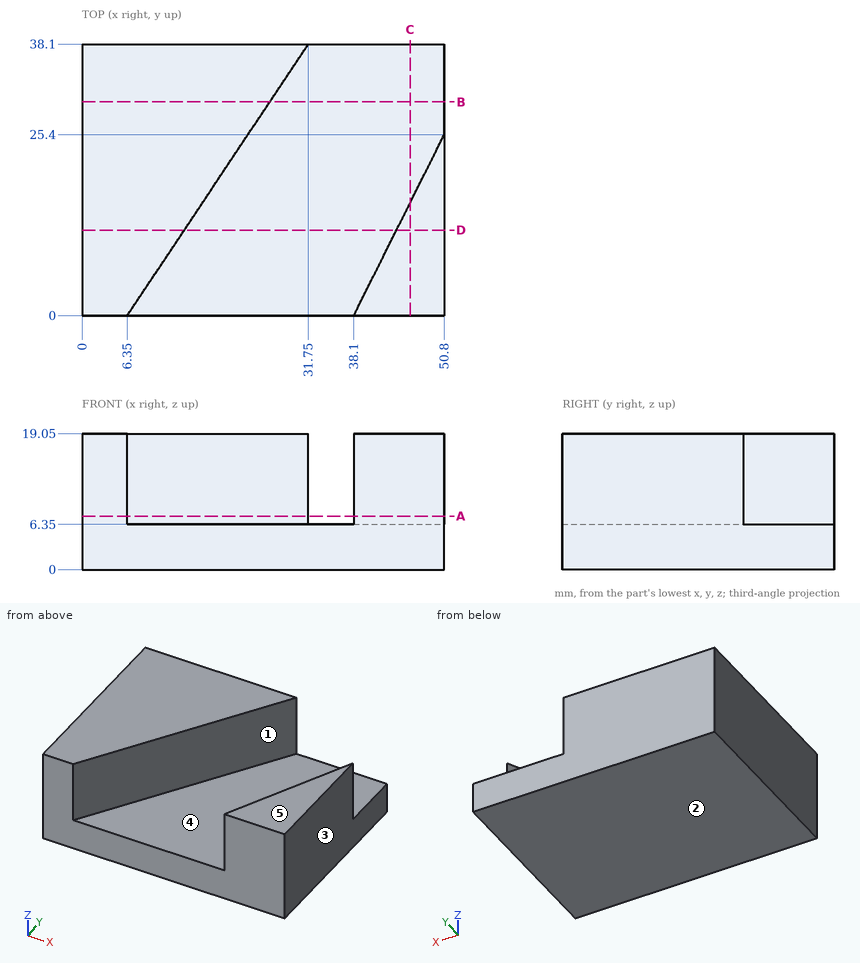
Verification items for this drawing (mm, ordinates from the low corner). A direction names the side the tool comes from. Coordinates: 2 decimals unless noted, no trailing zeros. Order: outer loops, then holes, each group sorted by start corner. A loop starts at its lowest first (then second) coordinate and runs counter-clockwise, first axis right, second up. Notation, with made-up numbers: (-23, 45) - (34, 45) arc R8 ccw to (34, 50) - close; hole circle Ø5 at (17, 70.5). An arc over 180 degrees is marked (long way). Use one line per item in the form item = value.
1. Access from +Z, -Z, +X, -X, +Y, -Y to the whole of each face (thin tool, end or side, straight path). Record for the marked faces 1 and 2.
Here are the results:
face_1 = +Z, -Y
face_2 = -Z, +X, -X, +Y, -Y
2. Gauge pin test, flat ends, axial feed: pin 1 (2 mm diameter, centred on x = 15.5, z = 11, fed in from -Y) (3 decimals); pin 2 (1.5 mm diameter, centred on x = 30.5, z = 9, fed in from -Y). Record the tip position at first contact, or that the pin passes through.
Here are the results:
pin_1 = 12.225
pin_2 = 35.1
3. Section check C-C (x = 46). Record the boundary of the cut face in (y, z), then the cut area to 3 significant figures.
Here are the results:
outline = (0, 0) - (38.1, 0) - (38.1, 6.35) - (15.8, 6.35) - (15.8, 19.05) - (0, 19.05) - close
area = 443 mm²
4. Section check D-D (y = 12). Record the boundary of the cut face in (x, z), then the cut area to 3 significant figures.
Here are the results:
outline = (0, 0) - (50.8, 0) - (50.8, 19.05) - (44.1, 19.05) - (44.1, 6.35) - (14.35, 6.35) - (14.35, 19.05) - (0, 19.05) - close
area = 590 mm²
5. Section check A-A (z = 7.5). Record the boundary of the cut face in (x, y).
Here are the results:
outline = (0, 0) - (6.35, 0) - (31.75, 38.1) - (0, 38.1) - close; (38.1, 0) - (50.8, 0) - (50.8, 25.4) - close
6. Draft check along X on the marked faces 3, 4 and 5. Enter one of: pulls with the +X half, pulls with the -X half, needs draft (parallel to the pull), parting line crosses it, or undercut.
Here are the results:
face_3 = pulls with the +X half
face_4 = undercut
face_5 = needs draft
7. Scan lines: line 1 (Z direction, x = 28, y = 13.5); line 2 (X direction, y = 14.5, z = 9). Record each from-to range of solid material in increasing order.
Here are the results:
line_1 = 0 to 6.35
line_2 = 0 to 16.02, 45.35 to 50.8
8. Section check B-B (y = 30). Record the boundary of the cut face in (x, z), then the cut area to 3 significant figures.
Here are the results:
outline = (0, 0) - (50.8, 0) - (50.8, 6.35) - (26.35, 6.35) - (26.35, 19.05) - (0, 19.05) - close
area = 657 mm²
